Here's how the part is built. I have some questions about the finished solid (model axes, mm). A direction names the side the tool comes from. Round coordinates to 2 decimals unless told otherwise and drop trailing zeros. Loops run counter-clockwise (first coordinate to the right, second up) from the corner with the lowest first, then second, coordinate; pieces in that order, holes last. Notation, with made-up numbers: M 31.5,-9 L 51.5,-9 A25 ccw 51.5,6 Z; hole C 46.25,78.25 d4. An arc over 180 degrees is marked long. Use a Markdown table: item, result.
```python
from build123d import *

# Parameters (mm, degrees)
SKETCH7_W           = 14.8
SKETCH7_H           = 103.2
BOSS_EXTRUDE4_DEPTH = 7
CUT_EXTRUDE2_DEPTH  = 15
LPATTERN1_COUNT     = 31
LPATTERN1_PITCH     = 3.44
SKETCH10_W          = 103.2
SKETCH10_H          = 2
BOSS_EXTRUDE5_DEPTH = 10.1
SKETCH11_W          = 103.2
SKETCH11_H          = 2
BOSS_EXTRUDE6_DEPTH = 10.1
SKETCH12_W          = 5.4
SKETCH12_H          = 5.4
CUT_EXTRUDE3_DEPTH  = 55.715719862


with BuildPart() as part:
    # Sketch7 → Boss-Extrude4 (new body)
    with BuildSketch(Plane.XY):
        Rectangle(SKETCH7_W, SKETCH7_H)
    extrude(amount=BOSS_EXTRUDE4_DEPTH)

    # Sketch9 → Cut-Extrude2 (cut)
    with BuildSketch(Plane.YZ.offset(7.4)):
        Polygon((-52.87, 7), (-52.051066973, 4.75), (-51.151066973, 4.75), (-50.332133946, 7), align=None)
    cut_extrude2 = extrude(amount=-CUT_EXTRUDE2_DEPTH, mode=Mode.SUBTRACT)

    # LPattern1: Cut-Extrude2 ×31
    with Locations(*[(0, i * LPATTERN1_PITCH, 0) for i in range(1, LPATTERN1_COUNT)]):
        add(cut_extrude2, mode=Mode.SUBTRACT)

    # Sketch10 → Boss-Extrude5 (add)
    with BuildSketch(Plane.YZ.offset(7.4)):
        with Locations((0, 1)):
            Rectangle(SKETCH10_W, SKETCH10_H)
    extrude(amount=BOSS_EXTRUDE5_DEPTH)

    # Sketch11 → Boss-Extrude6 (add)
    with BuildSketch(Plane(origin=(-7.4, 0, 0), x_dir=(0, -1, 0), z_dir=(-1, 0, 0))):
        with Locations((0, 1)):
            Rectangle(SKETCH11_W, SKETCH11_H)
    extrude(amount=BOSS_EXTRUDE6_DEPTH)

    # Sketch12 → Cut-Extrude3 (cut, through all)
    with BuildSketch(Plane.XY.offset(2)):
        with Locations((17.2, -41.9)):
            Rectangle(SKETCH12_W, SKETCH12_H)
        with Locations((17.2, 41.9)):
            Rectangle(SKETCH12_W, SKETCH12_H)
        with Locations((-17.2, 41.9)):
            Rectangle(SKETCH12_W, SKETCH12_H)
        with Locations((-17.2, -41.9)):
            Rectangle(SKETCH12_W, SKETCH12_H)
    extrude(amount=-CUT_EXTRUDE3_DEPTH, mode=Mode.SUBTRACT)


solid = part.part
```
Q1. I need wall thicknesses on line 1 (Y direction, x = 15, z = 1.5); line 2 (X direction, y = 44, z = 4.5); line 3 (Z direction, x = 15, y = 24.5). Which ranges of each line are inside material? Lowest first, please. Write a range as from..to.
Return value:
| item | result |
|---|---|
| line 1 | y = -51.6..-44.6, -39.2..39.2, 44.6..51.6 |
| line 2 | x = -7.4..7.4 |
| line 3 | z = 0..2 |
Q2. Imagine slicing it at A-A, the plane x = -12. Please give me the cut outline in (y, z).
Return value:
| item | result |
|---|---|
| outline | M -51.6,0 L 51.6,0 L 51.6,2 L -51.6,2 Z |
Q3. We'd pull the mould along Y, two halves only. Please class faces 1 (the flat face through (0, 51.6, 2)), 2 (the flat face through (-16, -39.2, 1)), 3 (the flat face through (-17.5, -48, 1)), 4 (the flat face through (0.104, -49.026, 5.891)): pulls with the +Y half, pulls with the -Y half, needs draft (parallel to the pull), parting line crosses it, or undercut.
Return value:
| item | result |
|---|---|
| face 1 | pulls with the +Y half |
| face 2 | undercut |
| face 3 | needs draft |
| face 4 | undercut |
Q4. Will these pins go through, and if not, where does the flat tip stop? P1, Ø5, axis at x = 11.5, y = 34.5, coming from the +Z side; P2, Ø1.5, axis at y = -14.5, z = 5, coming from the +X side.
Return value:
| item | result |
|---|---|
| P1 | stops at z = 2 |
| P2 | stops at x = 7.4 |
Q5. For faces 5 (the flat face through (0.104, -9.467, 5.859)), 6 (the flat face through (-12, 1, 2)), 7 (the flat face through (-14.5, -42, 1)), which set-ups out of +Z, -Z, +X, -X, +Y, -Y let a thin tool reach every point of the face, with its end or its side?
Return value:
| item | result |
|---|---|
| face 5 | +Z, +X, -X |
| face 6 | +Z, -X, +Y, -Y |
| face 7 | +Z, -Z, -X |
